Source: CAD feature listing. Evaluate the final solid. Frame: model axes, mm. Face numbers are marked on the shaded views. Coordinates: 2 decimals unless noted, no trailing zeros. Loops run counter-clockwise (first coordinate to the right, second up) from the corner with the lowest first, then second, coordinate; pieces in that order, holes last.
Item 1: Line query: probe 1 along X at (y, z) = (-25, 6.75); probe 2 along Z at (x, y) = (151, -5.5); probe 3 along Y at (x, z) = (112, 1.8). Output: solid intervals per line, ascending.
Item 2: Pull-direction query (Y, two-part tool) for the marked faces 1 and 2; classes: +Y half, -Y half, draft (parallel to the pull), parting line (faces both ways), or undercut.
Item 3: Section query C-C, the plane z = 3.5. Return the cut outline in (x, y), then the cut area to 3 significant figures.
Item 4: Section query D-D, the plane x = 68.5. Return the cut outline in (y, z), then the cut area to 3 significant figures.
Item 5: Section query B-B, the plane y = 0. Return the cut outline in (x, z), then the cut area to 3 significant figures.
Item 6: Pin query (flat end, axial travel): pin 1 Ø4 at (x, y) = (112, 0) entering from -Z; pin 2 Ø2 at (x, z) = (36, 19) entering from +Y; pin 3 Ø8 at (x, z) = (122.5, 9.5) entering from -Y; pin 4 Ø1 at (x, z) = (18.5, 11.5) entering from -Y. Return the tip coordinate at first contact, or that it passes through.
Item 7: Section query A-A, the plane x = 112. Return the cut outline in (y, z).
```python
from build123d import *

# Parameters (mm, degrees)
F1_DEPTH = 167
F3_D     = 6.6
F5_D     = 6.6


with BuildPart() as f1:
    # F0 (on Right) → F1 (new body)
    with BuildSketch(Plane.YZ):
        Polygon((-22.8742525516, 0), (20, 0), (20, 5), (-20, 5), (-30, 22.3205080757), (-34.1563406595, 19.5411498184), align=None)
    extrude(amount=F1_DEPTH)

    # F3 (through all)
    with Locations(Plane.XY.offset(5)):
        with Locations((112, 0), (55, 0)):
            Hole(F3_D / 2)

    # F5 (through all)
    with Locations(Plane(origin=(0, -17.1556894137, -9.9048419011), x_dir=(1, 0, 0), z_dir=(0, -0.8660254038, -0.5))):
        with Locations((20, 21.3301270189), (91, 21.3301270189), (157, 21.3301270189)):
            Hole(F5_D / 2)


solid = f1.part
```
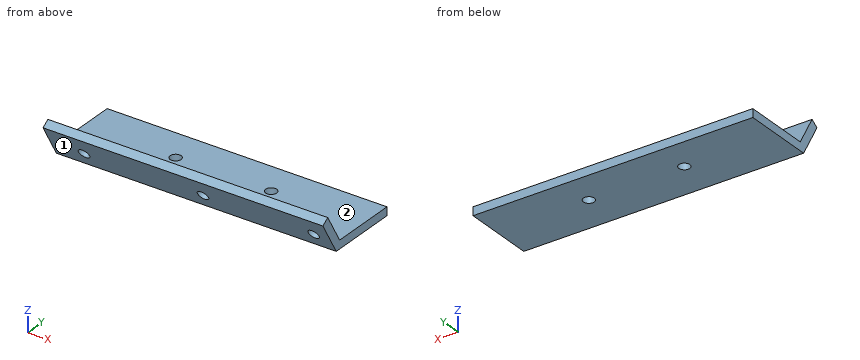
Verdict:
1. probe 1: x = 0 to 18.59, 21.41 to 89.59, 92.41 to 155.59, 158.41 to 167
1. probe 2: z = 0 to 5
1. probe 3: y = -23.91 to -3.3, 3.3 to 20
2. face 1: -Y half
2. face 2: draft
3. outline: (0, -24.89) - (167, -24.89) - (167, 20) - (0, 20) - close; hole circle Ø6.6 at (55, 0); hole circle Ø6.6 at (112, 0)
3. area: 7,430 mm2
4. outline: (-34.16, 19.54) - (-22.87, 0) - (20, 0) - (20, 5) - (-20, 5) - (-30, 22.32) - close
4. area: 313 mm2
5. outline: (0, 0) - (51.7, 0) - (51.7, 5) - (0, 5) - close; (58.3, 0) - (108.7, 0) - (108.7, 5) - (58.3, 5) - close; (115.3, 0) - (167, 0) - (167, 5) - (115.3, 5) - close
5. area: 769 mm2
6. pin 1: passes through
6. pin 2: stops at y = -27.51
6. pin 3: stops at y = -30.67
6. pin 4: stops at y = -29.8
7. outline: (-34.16, 19.54) - (-22.87, 0) - (-3.3, 0) - (-3.3, 5) - (-20, 5) - (-30, 22.32) - close; (3.3, 0) - (20, 0) - (20, 5) - (3.3, 5) - close
